from build123d import *

# Parameters (mm, degrees)
F1_DEPTH = 20
F2_R     = 10
F3_R     = 25
F5_D     = 10
F6_R     = 18
F7_DEPTH = 30
F9_D     = 14
F9_DEPTH = 31
F9_TIP   = 4.2060243332


with BuildPart() as f1:
    # F0 (on Top) → F1 (new body)
    with BuildSketch(Plane.XY):
        Polygon((0, 27.66993), (-58.33, 0), (0, -27.66993), (58.33, 0), align=None)
    extrude(amount=F1_DEPTH)

    # F2
    f2_edges = [f1.edges().sort_by_distance(p)[0] for p in [
        (-58.33, 0, 10),
        (58.33, 0, 10),
    ]]
    fillet(f2_edges, radius=F2_R)

    # F3
    f3_edges = [f1.edges().sort_by_distance(p)[0] for p in [
        (0, -27.66993, 10),
        (0, 27.66993, 10),
    ]]
    fillet(f3_edges, radius=F3_R)

    # F5 (through all)
    with Locations(Plane.XY.offset(20)):
        with Locations((34.9977554223, 0), (-34.9977554223, 0)):
            Hole(F5_D / 2)

    # F6 (on face) → F7 (join)
    with BuildSketch(Plane.XY.offset(20)):
        Circle(F6_R)
    extrude(amount=F7_DEPTH)

    # F9
    with Locations(Plane.XY.offset(50)):
        with Locations((0, 0)):
            Hole(F9_D / 2, depth=F9_DEPTH)
            with Locations((0, 0, -(F9_DEPTH + F9_TIP / 2))):  # 118° drill point
                Cone(0, F9_D / 2, F9_TIP, mode=Mode.SUBTRACT)


solid = f1.part
Design review of the part built by this model. Coordinates are the model's own, in mm. A direction names the side the tool comes from. Give positions to 0.01 mm unless a question says otherwise; leave off trailing zeros. Order: outer loops, then holes, each group sorted by start corner. A loop starts at its lowest first (then second) coordinate and runs counter-clockwise, first axis right, second up. Notation, with made-up numbers: (-23, 87.25) - (-14, 87.25) arc R29 cw to (-14, 110.25) - close; hole circle Ø2 at (44.25, 73.25). An arc over 180 degrees is marked (long way). Write item = value, one per line. Start each with the question number.
Q1. Clearance check with flat-ended pins moving along their axes: pin 1 Ø3 at (y, z) = (13.5, 23) entering from -X; pin 2 Ø12 at (x, z) = (-22.5, 39.5) entering from -Y; pin 3 Ø2 at (x, z) = (32, 6.5) entering from +Y. State where each tip first meets the part, or that it passes through.
Q2. We need section A-A on x = 33. State the section outline as (y, z) points, plus the area to 3 significant figures.
Q3. We need section B-B on z = 38.5. State the section outline as (x, y) points.
Q4. Mouldability with a two-part tool opening along Y and no side actions: class faces 3 (the face through (-2.343, 17.847, 34.79)), 4 (the face through (36.08, -4.88, 9.86)), 5 (the face through (0, -25, 10)) as released by +Y, released by -Y, zero draft, split by the parting line, or undercut.
Q5. To check wall thickness, follow L1, parallel to Y at x = 0, z = 42.5; L2, parallel to Z at x = 37, y = -10; L3, parallel to Y at x = -32, z = 10.5. State the ranges of each line that lie inside material, in increasing order. Write a range as from..to.
Q6. Tool access review of faces 1 (the face through (-44.997, 0.158, 10.14)), 2 (the face through (-6.466, -2.681, 34.283)): name each direction out of +Z, -Z, +X, -X, +Y, -Y from which nothing blocks a thin tool from reaching the whole face with its end or side.
Q7. We need section C-C on y = 12. State the section outline as (x, z) points, plus the area to 3 significant figures.
Q8. We need section D-D on x = 12. State the section outline as (y, z) points.
Working result:
q1.pin_1 = -13.42
q1.pin_2 = -7.19
q1.pin_3 = 12.96
q2.outline = (-12.02, 0) - (-4.58, 0) - (-4.58, 20) - (-12.02, 20) - close; (4.58, 0) - (12.02, 0) - (12.02, 20) - (4.58, 20) - close
q2.area = 297 mm²
q3.outline = circle Ø36 at (0, 0); hole circle Ø14 at (0, 0)
q4.face_3 = split by the parting line
q4.face_4 = undercut
q4.face_5 = released by -Y
q5.L1 = -18..-7, 7..18
q5.L2 = 0..20
q5.L3 = -12.49..-4, 4..12.49
q6.face_1 = +Z, -Z, -X
q6.face_2 = +Z
q7.outline = (-33.03, 0) - (33.03, 0) - (33.03, 20) - (13.42, 20) - (13.42, 50) - (-13.42, 50) - (-13.42, 20) - (-33.03, 20) - close
q7.area = 2,130 mm²
q8.outline = (-21.98, 0) - (21.98, 0) - (21.98, 20) - (13.42, 20) - (13.42, 50) - (-13.42, 50) - (-13.42, 20) - (-21.98, 20) - close
